Geometry check sheet. Reference: the model listing, model coordinates, mm. Face numbers are marked on the shaded views. Round coordinates to 2 decimals unless told otherwise and drop trailing zeros. Loops run counter-clockwise (first coordinate to the right, second up) from the corner with the lowest first, then second, coordinate; pieces in that order, holes last. Notation, with made-up numbers: (42.25, 7) -> (72.25, 7) arc R24 cw to (72.25, 35) -> close; hole circle Ø2 at (-30, 42.25). An arc over 180 degrees is marked (long way). Use a Markdown table: item, result. Add a question column.
Q1. Sectioned sample at D-D, the plane x = 171. Enter the section's corners in (y, z), then the cut area to 3 significant figures.
Q2. Sectioned sample at C-C, the plane z = -25.5. Enter the section's corners in (x, y).
Q3. Sectioned sample at B-B, the plane y = 34.5. Enter the section's corners in (x, z), then the cut area to 3 significant figures.
Q4. Release check for a two-part mould opening along Y. For the marked faces 1 and 2 record: released by +Y, released by -Y, zero draft, split by the parting line, or undercut.
Q5. Gauge pin test, flat ends, axial feed: P1, Ø4, axis at y = -89, z = -25, coming from the -X side; P2, Ø3, axis at x = 151, y = -47, coming from the +Z side; P3, Ø16, axis at x = -34.5, z = -9, coming from the +Y side; P4, Ø8.5, axis at x = -37, z = -15.5, coming from the +Y side. Record the tip position at first contact, or that the pin passes through.
Q6. Material ranges on L1, parallel to Y at x = 49.5, z = -14.5; L2, parallel to Z at x = -46, y = -88; L3, parallel to X at y = 62, z = -21, recorded low to high.
Q7. Sectioned sample at A-A, the plane x = -122. Enter the section's corners in (y, z), then the cut area to 3 significant figures.
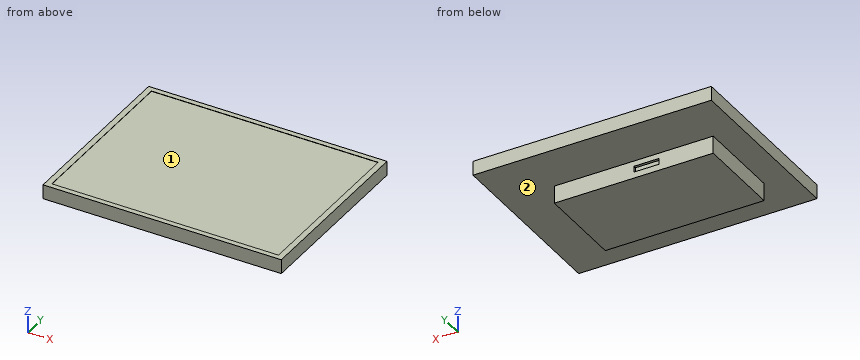
```python
from build123d import *

# Parameters (mm, degrees)
F0_W     = 435
F0_H     = 332
F1_DEPTH = 26
F2_W     = 413.8
F2_H     = 313
F3_DEPTH = 0.5
F4_W     = 290
F4_H     = 160
F5_DEPTH = 32
F6_W     = 45.65622
F6_H     = 10.88232
F7_DEPTH = 5


with BuildPart() as f1:
    # F0 (on Top) → F1 (new body)
    with BuildSketch(Plane.XY):
        Rectangle(F0_W, F0_H)
    extrude(amount=F1_DEPTH)

    # F2 (on face) → F3 (cut)
    with BuildSketch(Plane.XY.offset(26)):
        Rectangle(F2_W, F2_H)
    extrude(amount=-F3_DEPTH, mode=Mode.SUBTRACT)

    # F4 (on face) → F5 (join)
    with BuildSketch(Plane.XY):
        with Locations((-22.5, -6)):
            Rectangle(F4_W, F4_H)
    extrude(amount=-F5_DEPTH)

    # F6 (on face) → F7 (cut)
    with BuildSketch(Plane(origin=(0, 74, 0), x_dir=(-1, 0, 0), z_dir=(0, 1, 0))):
        with Locations((45.32811, -15.279424)):
            Rectangle(F6_W, F6_H)
    extrude(amount=-F7_DEPTH, mode=Mode.SUBTRACT)


solid = f1.part
```
Values:
| question | item | result |
|---|---|---|
| 1 | outline | (-166, 0) -> (166, 0) -> (166, 26) -> (156.5, 26) -> (156.5, 25.5) -> (-156.5, 25.5) -> (-156.5, 26) -> (-166, 26) -> close |
| 1 | area | 8,480 mm^2 |
| 2 | outline | (-167.5, -86) -> (122.5, -86) -> (122.5, 74) -> (-167.5, 74) -> close |
| 3 | outline | (-217.5, 0) -> (-167.5, 0) -> (-167.5, -32) -> (122.5, -32) -> (122.5, 0) -> (217.5, 0) -> (217.5, 26) -> (206.9, 26) -> (206.9, 25.5) -> (-206.9, 25.5) -> (-206.9, 26) -> (-217.5, 26) -> close |
| 3 | area | 20,400 mm^2 |
| 4 | face 1 | undercut |
| 4 | face 2 | zero draft |
| 5 | P1 | through |
| 5 | P2 | z = 25.5 |
| 5 | P3 | y = 74 |
| 5 | P4 | y = 69 |
| 6 | L1 | -86 to 74 |
| 6 | L2 | 0 to 25.5 |
| 6 | L3 | -167.5 to 122.5 |
| 7 | outline | (-166, 0) -> (-86, 0) -> (-86, -32) -> (74, -32) -> (74, 0) -> (166, 0) -> (166, 26) -> (156.5, 26) -> (156.5, 25.5) -> (-156.5, 25.5) -> (-156.5, 26) -> (-166, 26) -> close |
| 7 | area | 13,600 mm^2 |
